For this review, take the finished solid that the model builds, in its own axes (mm). A direction names the side the tool comes from. Give positions to 0.01 mm unless a question says otherwise; leave off trailing zeros. Order: outer loops, then holes, each group sorted by start corner. A loop starts at its lowest first (then second) coordinate and runs counter-clockwise, first axis right, second up.
Item 1: For P1, Ø6, axis at y = 21, z = -2, coming from the -X side; P2, Ø1.3, axis at y = 1, z = -21, coming from the +X side; P3, Ø1.3, axis at x = 13, y = 2, coming from the -Z side, all flat-tipped, find the tip position at first contact; note any pin that passes through.
Item 2: For probe 1 along Z at (x, y) = (10.5, 8); probe 2 along Z at (x, y) = (14.75, 5.5); probe 3 along Y at (x, z) = (13.75, -9.5), list the stretches that pass through material, from the lowest coordinate up.
Item 3: Machinability: for faces 1 (the flat face through (0, 5, -7)), 2 (the flat face through (14, 5, 60.062)), 3 (the flat face through (5.75, 5, 60)), 4 (the flat face through (10, 1, -14)), which of the approach directions +Z, -Z, +X, -X, +Y, -Y give a long, thin tool a straight path to every point of the face, cutting with its end or side? Answer none if there is none.
Item 4: The part is to be moulded in two halves that separate along Y. For faces 5 (the flat face through (9, 5, 62.062)), 6 (the flat face through (7, -20.443, -7)), 7 (the flat face through (13, -1.443, -14)), say which applies: released by +Y, released by -Y, zero draft, split by the parting line, or undercut.
Item 5: Consider section A-A (z = 37). Give the boundary of the cut face in (x, y).
Item 6: Consider section B-B (y = 22). Give the boundary of the cut face in (x, z).
```python
from build123d import *

# Parameters (mm, degrees)
SKETCH1_W           = 145
SKETCH1_H           = 51
BOSS_EXTRUDE1_DEPTH = 15
CUT_EXTRUDE3_DEPTH  = 52
SKETCH7_W           = 5
SKETCH7_H           = 4.5
CUT_EXTRUDE5_DEPTH  = 135


with BuildPart() as part:
    # Sketch1 → Boss-Extrude1 (new body)
    with BuildSketch(Plane(origin=(0, 0, 0), x_dir=(0, 0, -1), z_dir=(1, 0, 0))):
        with Locations((7.937921078, 5.057266603)):
            Rectangle(SKETCH1_W, SKETCH1_H)
    extrude(amount=BOSS_EXTRUDE1_DEPTH)

    # Sketch6 → Cut-Extrude3 (cut, through all)
    with BuildSketch(Plane(origin=(0, 30.557266603, 0), x_dir=(1, 0, 0), z_dir=(0, 1, 0))):
        Polygon((12.5, -60.062078922), (15, -60.062078922), (15, -57.062078922), (12.5, -57.062078922), (5.75, -57.062078922), (5.75, -62.062078922), (12.5, -62.062078922), align=None)
    extrude(amount=-CUT_EXTRUDE3_DEPTH, mode=Mode.SUBTRACT)

    # Sketch7 → Cut-Extrude5 (cut)
    with BuildSketch(Plane(origin=(0, 0, -80.437921078), x_dir=(-1, 0, 0), z_dir=(0, 0, -1))):
        with Locations((-12.5, 0.807266603)):
            Rectangle(SKETCH7_W, SKETCH7_H)
    extrude(amount=-CUT_EXTRUDE5_DEPTH, mode=Mode.SUBTRACT)


solid = part.part
```
Resolved:
1. P1: stops at x = 0
1. P2: stops at x = 10
1. P3: stops at z = 54.56
2. probe 1: z = -80.44 to 57.06, 62.06 to 64.56
2. probe 2: z = -80.44 to 57.06, 60.06 to 64.56
2. probe 3: y = -20.44 to -1.44, 3.06 to 30.56
3. face 1: +Z, -Z, -X, +Y, -Y
3. face 2: +X, +Y, -Y
3. face 3: +Y, -Y
3. face 4: -Z, +X
4. face 5: zero draft
4. face 6: released by -Y
4. face 7: undercut
5. outline: (0, -20.44) - (15, -20.44) - (15, -1.44) - (10, -1.44) - (10, 3.06) - (15, 3.06) - (15, 30.56) - (0, 30.56) - close
6. outline: (0, -80.44) - (15, -80.44) - (15, 57.06) - (5.75, 57.06) - (5.75, 62.06) - (12.5, 62.06) - (12.5, 60.06) - (15, 60.06) - (15, 64.56) - (0, 64.56) - close
